from build123d import *

# Parameters (mm, degrees)
SKETCH_1_W          = 6.6
SKETCH_1_H          = 54
SKETCH_1_R          = 1.49999954
EXTRUDE_1_DEPTH     = 12
FILLET_1_R          = 6
SKETCH_2_W          = 34
SKETCH_2_H          = 14
CUT_EXTRUDE_1_DEPTH = 20
FILLET_2_R          = 2
SKETCH_3_W          = 1
SKETCH_3_H          = 2.5
CUT_EXTRUDE_2_DEPTH = 31.274742098
SKETCH_4_W          = 14.557801868
SKETCH_4_H          = 48.8
CUT_EXTRUDE_3_DEPTH = 2
SKETCH_6_R          = 1.5
SKETCH_6_R_2        = 1
SKETCH_6_R_3        = 1.49999954
EXTRUDE_2_DEPTH     = 4


with BuildPart() as part:
    # 草图1 → 凸台-拉伸1 (new body)
    with BuildSketch(Plane(origin=(0, 0, 0), x_dir=(1, 0, 0), z_dir=(0, 1, 0))):
        with Locations((-25, 0)):
            Rectangle(SKETCH_1_W, SKETCH_1_H)
        with Locations(Location((-25, -21.49999992, 0), (0, 0, 270))):
            Circle(SKETCH_1_R, mode=Mode.SUBTRACT)
        with Locations(Location((-25, 20.9999989, 0), (0, 0, 270))):
            Circle(SKETCH_1_R, mode=Mode.SUBTRACT)
    extrude(amount=EXTRUDE_1_DEPTH)

    # 圆角1
    # the kernel refuses this fillet: 6 mm, written as the material it takes off along each edge
    with BuildSketch(Plane(origin=(-6.7, 12, 27), x_dir=(0, -1, 0), z_dir=(-1, 0, 0)), Plane(origin=(-43.3, 12, -27), x_dir=(0, -1, 0), z_dir=(1, 0, 0))) as fillet_1_piece_1:
        with BuildLine():
            CenterArc((FILLET_1_R, -FILLET_1_R), FILLET_1_R, 90, 90)
            Line((0, -FILLET_1_R), (0, 0))
            Line((0, 0), (FILLET_1_R, 0))
        make_face()
    extrude(amount=36.6, mode=Mode.SUBTRACT)

    # 草图2 → 切除-拉伸1 (cut)
    with BuildSketch(Plane.ZY.offset(28.3)):
        Rectangle(SKETCH_2_W, SKETCH_2_H)
    extrude(amount=-CUT_EXTRUDE_1_DEPTH, mode=Mode.SUBTRACT)

    # 圆角2
    fillet_2_edges = [part.edges().sort_by_distance(p)[0] for p in [
        (-25, 7, 17),
        (-25, 7, -17),
    ]]
    fillet(fillet_2_edges, radius=FILLET_2_R)

    # 草图3 → 切除-拉伸2 (cut, through all)
    with BuildSketch(Plane.ZY.offset(28.3)):
        with Locations((0, 10.75)):
            Rectangle(SKETCH_3_W, SKETCH_3_H)
        with Locations((4, 10.75)):
            Rectangle(SKETCH_3_W, SKETCH_3_H)
        with Locations((8, 10.75)):
            Rectangle(SKETCH_3_W, SKETCH_3_H)
        with Locations((12, 10.75)):
            Rectangle(SKETCH_3_W, SKETCH_3_H)
        with Locations((16, 10.75)):
            Rectangle(SKETCH_3_W, SKETCH_3_H)
        with Locations((20, 10.75)):
            Rectangle(SKETCH_3_W, SKETCH_3_H)
        with Locations((-4, 10.75)):
            Rectangle(SKETCH_3_W, SKETCH_3_H)
        with Locations((-8, 10.75)):
            Rectangle(SKETCH_3_W, SKETCH_3_H)
        with Locations((-12, 10.75)):
            Rectangle(SKETCH_3_W, SKETCH_3_H)
        with Locations((-16, 10.75)):
            Rectangle(SKETCH_3_W, SKETCH_3_H)
        with Locations((-20, 10.75)):
            Rectangle(SKETCH_3_W, SKETCH_3_H)
    extrude(amount=-CUT_EXTRUDE_2_DEPTH, mode=Mode.SUBTRACT)

    # 草图4 → 切除-拉伸3 (cut)
    with BuildSketch(Plane.XZ):
        with Locations((-25, 0.25000051)):
            Rectangle(SKETCH_4_W, SKETCH_4_H)
    extrude(amount=-CUT_EXTRUDE_3_DEPTH, mode=Mode.SUBTRACT)

    # 草图6 → 凸台-拉伸2 (add)
    # profile 1 of 2: a face of its own
    with BuildSketch(Plane.XZ.offset(-2)):
        with Locations(Location((-25, 21.49999992, 0), (0, 0, 270))):
            Circle(SKETCH_6_R)
        with Locations(Location((-25, 21.49999992, 0), (0, 0, 270))):
            Circle(SKETCH_6_R_2, mode=Mode.SUBTRACT)
    # profile 2 of 2: a face of its own
    with BuildSketch(Plane.XZ.offset(-2)):
        with Locations(Location((-25, -20.9999989, 0), (0, 0, 270))):
            Circle(SKETCH_6_R_3)
        with Locations(Location((-25, -20.9999989, 0), (0, 0, 270))):
            Circle(SKETCH_6_R_2, mode=Mode.SUBTRACT)
    extrude(amount=-EXTRUDE_2_DEPTH)


solid = part.part
The listing builds one solid part. Answer for the finished solid, in the listing's coordinates (mm). A direction names the side the tool comes from. Give positions to 0.01 mm unless a question says otherwise; leave off trailing zeros. Order: outer loops, then holes, each group sorted by start corner. A loop starts at its lowest first (then second) coordinate and runs counter-clockwise, first axis right, second up. Notation, with made-up numbers: (42.25, 35) -> (96.25, 35) arc R20 ccw to (96.25, 51) -> close; hole circle Ø4 at (36, 53). An arc over 180 degrees is marked (long way). Put each result on its own line as item: value.
Item 1: For faces 4 (the face through (-25, 0, 26)), 5 (the face through (-24.95, 6.4, 16.43)), 6 (the face through (-23, 9.5, -20)), determine the directions among +Z, -Z, +X, -X, +Y, -Y from which every point of the face is accessible in a straight line to the end or side of a thin tool.
Established:
face 4: +Z, -Z, +X, -X, -Y
face 5: +X, -X, -Y
face 6: +X, -X, +Y
Item 2: A cutting plane is placed at D-D on z = 1. Give the vertices of the cut face in (x, y), plus the area to 3 significant figures.
Established:
outline: (-28.3, 7) -> (-21.7, 7) -> (-21.7, 12) -> (-28.3, 12) -> close
area: 33.0 mm^2
Item 3: A cutting plane is placed at C-C on y = 9. Give the vertices of the cut face in (x, z).
Established:
outline: (-28.3, -26.2) -> (-21.7, -26.2) -> (-21.7, 26.2) -> (-28.3, 26.2) -> close; hole circle Ø3 at (-25, -21); hole circle Ø3 at (-25, 21.5)
Item 4: A cutting plane is placed at B-B on z = 21.5. Give the vertices of the cut face in (x, y), plus the area to 3 significant figures.
Established:
outline: (-28.3, 2) -> (-26, 2) -> (-26, 6) -> (-26.5, 6) -> (-26.5, 11.98) -> (-28.3, 11.98) -> close; (-24, 2) -> (-21.7, 2) -> (-21.7, 11.98) -> (-23.5, 11.98) -> (-23.5, 6) -> (-24, 6) -> close
area: 39.9 mm^2
Item 5: A cutting plane is placed at A-A on y = 3. Give the vertices of the cut face in (x, z).
Established:
outline: (-28.3, -27) -> (-21.7, -27) -> (-21.7, -17) -> (-28.3, -17) -> close; (-28.3, 17) -> (-21.7, 17) -> (-21.7, 27) -> (-28.3, 27) -> close; hole circle Ø2 at (-25, -21); hole circle Ø2 at (-25, 21.5)
Item 6: For a pull along Z with two mould halves and no side action, classify faces 1 (the face through (-25.046, 10.196, -25.289)), 2 (the face through (-25, 12, -18)), 3 (the face through (-25, 11, 19.5)) as released by +Z, released by -Z, zero draft, split by the parting line, or undercut.
Established:
face 1: released by -Z
face 2: zero draft
face 3: undercut
Item 7: Given P1, Ø0.8, axis at x = -24, y = 10.5, coming from the -Z side; P2, Ø3, axis at x = -25, y = 10, coming from the +Z side; P3, Ø0.8, axis at x = -27, y = 11, coming from the -Z side, each flat-ended and moving along its own axis, determine where each tip first touches the part or whether it passes through.
Established:
P1: stops at z = -25.38
P2: stops at z = 26.45
P3: stops at z = -24.85
Item 8: Straight lines are drawn through the part: line 1 (X direction, y = 3.1, z = 21.5); line 2 (X direction, y = 7.5, z = 21.5); line 3 (Z direction, x = -24.5, y = 7.25). For each, find the intervals that lie inside material, in ascending order.
Established:
line 1: x = -28.3 to -26, -24 to -21.7
line 2: x = -28.3 to -26.5, -23.5 to -21.7
line 3: z = -26.87 to -22.41, -19.59 to 20.09, 22.91 to 26.87
